from build123d import *

# Parameters (mm, degrees)
SKETCH_1_W          = 85
SKETCH_1_H          = 56
EXTRUDE_1_DEPTH     = 5
SKETCH_2_W          = 33
SKETCH_2_H          = 5
EXTRUDE_2_DEPTH     = 13
SKETCH_3_W          = 70
SKETCH_3_H          = 51
SKETCH_3_W_2        = 68
SKETCH_3_H_2        = 49
CUT_EXTRUDE_1_DEPTH = 1


with BuildPart() as part:
    # Эскиз1 → Бобышка-Вытянуть1 (new body)
    with BuildSketch(Plane(origin=(0, 0, 0), x_dir=(1, 0, 0), z_dir=(0, 1, 0))):
        with Locations((42.5, 28)):
            Rectangle(SKETCH_1_W, SKETCH_1_H)
    extrude(amount=EXTRUDE_1_DEPTH)

    # Эскиз2 → Бобышка-Вытянуть2 (add)
    with BuildSketch(Plane(origin=(0, 5, 0), x_dir=(1, 0, 0), z_dir=(0, 1, 0))):
        with Locations((23.5, 3.5)):
            Rectangle(SKETCH_2_W, SKETCH_2_H)
    extrude(amount=EXTRUDE_2_DEPTH)

    # Эскиз3 → Вырез-Вытянуть-Тонкостенный1 (cut)
    with BuildSketch(Plane.XZ):
        with Locations((41.5, -29)):
            Rectangle(SKETCH_3_W, SKETCH_3_H)
        with Locations((41.5, -29)):
            Rectangle(SKETCH_3_W_2, SKETCH_3_H_2, mode=Mode.SUBTRACT)
    extrude(amount=-CUT_EXTRUDE_1_DEPTH, mode=Mode.SUBTRACT)


solid = part.part
Source: CAD feature listing. Evaluate the final solid. Frame: model axes, mm. A direction names the side the tool comes from. Coordinates: 2 decimals unless noted, no trailing zeros. Order: outer loops, then holes, each group sorted by start corner. A loop starts at its lowest first (then second) coordinate and runs counter-clockwise, first axis right, second up. Notation, with made-up numbers: M 83.25,-21 L 133.25,-21 A22 ccw 133.25,17 Z; hole C -22,57 d8. An arc over 180 degrees is marked long. Write each question's results on one line, items separated by ' | '. Start each with the question number.
Item 1: Cut plane A-A (x = 20.5). Return loops of the section in (y, z), and give its area (3 significant figures).
Item 2: Set-up query: faces 1 (the face through (85, 2, -28)), 2 (the face through (40, 11, -3)), 3 (the face through (7, 11, -3)). Return all of +Z, -Z, +X, -X, +Y, -Y with unobstructed straight access to the full face (end or side cutting, diameter ignored); none if empty.
Item 3: Line query: probe 1 along Y at (x, z) = (52.5, -11.5); probe 2 along Z at (x, y) = (30, 6.5); probe 3 along X at (y, z) = (5.25, -2.5). Output: solid intervals per line, ascending.
Item 4: Cut plane B-B (z = -25). Return loops of the section in (x, y), and give its area (3 significant figures).
Item 5: First-contact query: pin 1 Ø10 at (y, z) = (4, -49) entering from -X; pin 2 Ø2 at (y, z) = (10.5, -6) entering from -X; pin 3 Ø10.5 at (x, y) = (18.5, 12) entering from +Z; pin 4 Ø2.5 at (y, z) = (14, -4.5) entering from +X. Flat tips, straight axial feed; report the tip coordinate or a pass-through.
Item 6: Cut plane D-D (x = 73.5). Return loops of the section in (y, z).
Item 7: Draft query along Z for faces 4 (the face through (23, 11, -6)), 5 (the face through (23, 11, -1)), 6 (the face through (23, 18, -4)), 7 (the face through (41, 1, -4)). Return one class per face: pulls with the +Z half, pulls with the -Z half, needs draft (parallel to the pull), parting line crosses it, or undercut.
Item 8: Cut plane C-C (y = 13). Return loops of the section in (x, z).
Checked values:
1) outline: M 0,-56 L 5,-56 L 5,-6 L 18,-6 L 18,-1 L 5,-1 L 5,0 L 0,0 L 0,-3.5 L 1,-3.5 L 1,-4.5 L 0,-4.5 L 0,-53.5 L 1,-53.5 L 1,-54.5 L 0,-54.5 Z | area: 343 mm2
2) face 1: +Z, -Z, +X, +Y, -Y | face 2: +Z, -Z, +X, +Y | face 3: +Z, -Z, -X, +Y
3) probe 1: y = 0 to 5 | probe 2: z = -6 to -1 | probe 3: x = 7 to 40
4) outline: M 0,0 L 6.5,0 L 6.5,1 L 7.5,1 L 7.5,0 L 75.5,0 L 75.5,1 L 76.5,1 L 76.5,0 L 85,0 L 85,5 L 0,5 Z | area: 423 mm2
5) pin 1: stops at x = 0 | pin 2: stops at x = 7 | pin 3: stops at z = -1 | pin 4: stops at x = 40
6) outline: M 0,-56 L 5,-56 L 5,0 L 0,0 L 0,-3.5 L 1,-3.5 L 1,-4.5 L 0,-4.5 L 0,-53.5 L 1,-53.5 L 1,-54.5 L 0,-54.5 Z
7) face 4: pulls with the -Z half | face 5: pulls with the +Z half | face 6: needs draft | face 7: undercut
8) outline: M 7,-6 L 40,-6 L 40,-1 L 7,-1 Z
